Can you work these out from the model? Positions are in its coordinate system, mm. Round coordinates to 2 decimals unless told otherwise and drop trailing zeros. Write each loop counter-clockwise with the first axis right and the second up, starting at its lowest first coordinate (ties: lowest second). Pieces come first, ordered by that corner, then holes. Notation, with made-up numbers: (6, -39) -> (64, -39) arc R11 cw to (64, -19) -> close; hole circle Ø7 at (-31, -7). An arc over 180 degrees is marked (long way). Use CSV: the item, a comma, the result in double quotes.
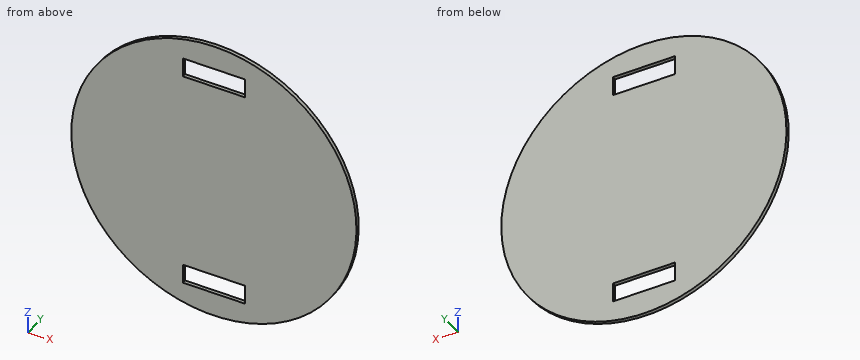
```python
from build123d import *

# Parameters (mm, degrees)
ESQUISSE2_R             = 150
BOSS_EXTRU_1_DEPTH      = 4
ESQUISSE4_W             = 65
ESQUISSE4_H             = 20
ENL_V_MAT_EXTRU_1_DEPTH = 213.169743366


with BuildPart() as part:
    # Esquisse2 → Boss.-Extru.1 (new body)
    with BuildSketch(Plane(origin=(0, 0, 0), x_dir=(1, 0, 0), z_dir=(0, 1, 0))):
        with Locations(Location((0, 0, 0), (0, 0, 270))):
            Circle(ESQUISSE2_R)
    extrude(amount=-BOSS_EXTRU_1_DEPTH)

    # Esquisse4 → Enlèv. mat.-Extru.1 (cut, through all)
    with BuildSketch(Plane(origin=(0, 0, 0), x_dir=(1, 0, 0), z_dir=(0, 1, 0))):
        with Locations((0, -115)):
            Rectangle(ESQUISSE4_W, ESQUISSE4_H)
        with Locations((0, 115)):
            Rectangle(ESQUISSE4_W, ESQUISSE4_H)
    extrude(amount=-ENL_V_MAT_EXTRU_1_DEPTH, mode=Mode.SUBTRACT)


solid = part.part
```
Q1. Suppose I cut it at B-B (x = 0). Write out the boundary of the cut face in (y, z), and give its area (3 significant figures).
Resolved:
outline,"(-4, -150) -> (0, -150) -> (0, -125) -> (-4, -125) -> close; (-4, -105) -> (0, -105) -> (0, 105) -> (-4, 105) -> close; (-4, 125) -> (0, 125) -> (0, 150) -> (-4, 150) -> close"
area,"1,040 mm^2"
Q2. Suppose I cut it at D-D (x = 81.5). Write out the boundary of the cut face in (y, z).
Resolved:
outline,"(-4, -125.93) -> (0, -125.93) -> (0, 125.93) -> (-4, 125.93) -> close"
Q3. Please list where these lines run through material, in increasing order: probe 1 along Z at (x, y) = (-16, -3.3); probe 2 along Z at (x, y) = (13.5, -1.95); probe 3 along X at (y, z) = (-0.45, 1.5).
Resolved:
probe 1,"z = -149.14 to -125, -105 to 105, 125 to 149.14"
probe 2,"z = -149.39 to -125, -105 to 105, 125 to 149.39"
probe 3,"x = -149.99 to 149.99"
Q4. Suppose I cut it at A-A (y = -3.1). Write out the boundary of the cut face in (x, z).
Resolved:
outline,"circle Ø300 at (0, 0); hole (-32.5, -125) -> (32.5, -125) -> (32.5, -105) -> (-32.5, -105) -> close; hole (-32.5, 105) -> (32.5, 105) -> (32.5, 125) -> (-32.5, 125) -> close"
Q5. Suppose I cut it at C-C (z = 114). Write out the boundary of the cut face in (x, y), and give its area (3 significant figures).
Resolved:
outline,"(-97.49, -4) -> (-32.5, -4) -> (-32.5, 0) -> (-97.49, 0) -> close; (32.5, -4) -> (97.49, -4) -> (97.49, 0) -> (32.5, 0) -> close"
area,"520 mm^2"
Q6. Will these pins go through, and if not, where does the flat tip stop? P1, Ø2, axis at x = -40.5, y = -2, coming from the +Z side; P2, Ø1.2, axis at y = -2.5, z = -114, coming from the -X side; P3, Ø1.2, axis at x = -1, y = -1, coming from the -Z side; P4, Ø1.2, axis at x = -0.5, y = -1.5, coming from the +Z side.
Resolved:
P1,"stops at z = 144.71"
P2,"stops at x = -98.19"
P3,"stops at z = -150"
P4,"stops at z = 150"
